Part model, mm, in its own coordinate system. Round coordinates to 2 decimals unless told otherwise and drop trailing zeros. Order: outer loops, then holes, each group sorted by start corner. A loop starts at its lowest first (then second) coordinate and runs counter-clockwise, first axis right, second up. Notation, with made-up numbers: (-15, 15) - (-9, 15) arc R31 ccw to (-9, 52) - close; hole circle Ø10 at (17.5, 35.25). An arc over 180 degrees is marked (long way). Return JSON: item names as keys, results as strings. Group by question number.
Item 1: Saw through at B-B on z = 0.9. State how many separate pieces and enclosed holes the cut face has, and give its area (3 significant figures).
Item 2: Saw through at A-A on x = 292. List the corners of the cut face in (y, z) (3 decimals), and give its area (3 significant figures).
Item 3: Drop flat-ended pins along their axis: pin 1 (1 mm diameter, centred on y = 36.5, z = 2, fed in from +X); pin 2 (6.5 mm diameter, centred on x = 660.4, y = 9.525, fed in from -Z). Give the stop position or say it passes through.
Item 4: Probe probe 1 along Y at (x, z) = (190.5, 1.4); probe 2 along Y at (x, z) = (469.9, 1.3); probe 3 along X at (y, z) = (43.5, 1.95). List the from-to ranges inside material, lowest first.
Item 5: Two-plate mould, pull along X, no slides. Class faces 1 (the face through (838.38, 19.32, 1.61)), 2 (the face through (431, 50, 0)), 3 (the face through (743.7, 40.3, 1.6)): released by +X, released by -X, zero draft, split by the parting line, or undercut.
Autodesk Inventor part; units mm, degrees
ref_plane "YZ Plane" through (0, 0, 0) normal (1, 0, 0) x (0, 1, 0)
ref_plane "XZ Plane" through (0, 0, 0) normal (0, 1, 0) x (-1, 0, 0)
ref_plane "XY Plane" through (0, 0, 0) normal (0, 0, 1) x (1, 0, 0)
sketch "Sketch1" plane through (0, 0, 0) normal (0, 0, 1) x (1, 0, 0)
  line L0 (0, 0) -> (850.9, 0)
  line L1 (850.9, 0) -> (850.9, 76.2)
  line L2 (850.9, 76.2) -> (0, 76.2)
  line L3 (0, 76.2) -> (0, 0)
  dimension "d0" = 850.9
  dimension "d1" = 76.2
extrude "Extrusion1" add sketch "Sketch1" along normal blind 3.175
sketch "Sketch4" plane through (0, 0, 3.175) normal (0, 0, 1) x (1, 0, 0)
  line L0 (0, 0) -> (0, 38.1)
  line L1 (0, 76.2) -> (0, 0)
  line L2 (0, 0) -> (25.4, 0)
  line L3 (0, 0) -> (850.9, 0)
  line L4 (25.4, 0) -> (0, 38.1)
  line L5 (850.9, 0) -> (825.5, 0)
  line L6 (850.9, 0) -> (850.9, 38.1)
  line L7 (850.9, 0) -> (850.9, 76.2)
  line L8 (850.9, 38.1) -> (825.5, 0)
  line L9 (0, 38.1) -> (0, 36.5125)
  circle A0 centre (292.9509, 36.5125) radius 14.2875
  circle A1 centre (557.9491, 36.5125) radius 14.2875
  circle A2 centre (757.9743, 39.6875) radius 14.2875
  circle A3 centre (92.9257, 39.6875) radius 14.2875
  dimension "d24" = 38.1
  dimension "d26" = 25.4
  dimension "d27" = 38.1
  dimension "d33" = 28.575
  dimension "d34" = 28.575
  dimension "d38" = 28.575
  dimension "d39" = 28.575
extrude "Extrusion3" cut sketch "Sketch4" against normal blind 3.175
sketch "Sketch5" plane through (0, 0, 3.175) normal (0, 0, 1) x (1, 0, 0)
  line L0 (850.9, 76.2) -> (0, 76.2)
  line L1 (0, 76.2) -> (425.45, 76.2)
  circle A0 centre (425.45, 66.675) radius 3.5687
  circle A1 centre (425.45, 9.525) radius 3.5687
  line L2 (25.4, 0) -> (825.5, 0)
  line L3 (0, 76.2) -> (190.5, 76.2)
  circle A2 centre (190.5, 66.675) radius 3.5687
  circle A3 centre (190.5, 9.525) radius 3.5687
  circle A4 centre (190.5, 38.1) radius 3.5687
  line L4 (850.9, 38.1) -> (850.9, 76.2)
  line L5 (850.9, 76.2) -> (660.4, 76.2)
  circle A5 centre (660.4, 66.675) radius 3.5687
  circle A6 centre (660.4, 9.525) radius 3.5687
  circle A7 centre (660.4, 38.1) radius 3.5687
  circle A8 centre (838.2, 63.5) radius 3.5687
  circle A9 centre (12.7, 63.5) radius 3.5687
  line L6 (0, 76.2) -> (0, 38.1)
  circle A10 centre (34.925, 12.7) radius 3.5687
  circle A11 centre (815.975, 12.7) radius 3.5687
  point P0 (0, 0)
  dimension "d42" = 425.45
  dimension "d43" = 7.1374
  dimension "d44" = 9.525
  dimension "d45" = 7.1374
  dimension "d46" = 9.525
  dimension "d47" = 190.5
  dimension "d48" = 7.1374
  dimension "d49" = 9.525
  dimension "d50" = 7.1374
  dimension "d51" = 9.525
  dimension "d52" = 7.1374
  dimension "d53" = 38.1
  dimension "d54" = 190.5
  dimension "d55" = 7.1374
  dimension "d56" = 9.525
  dimension "d57" = 7.1374
  dimension "d58" = 9.525
  dimension "d59" = 7.1374
  dimension "d60" = 38.1
  dimension "d61" = 7.1374
  dimension "d62" = 12.7
  dimension "d63" = 12.7
  dimension "d64" = 7.1374
  dimension "d65" = 12.7
  dimension "d66" = 12.7
  dimension "d67" = 7.1374
  dimension "d69" = 12.7
  dimension "d70" = 9.525
  dimension "d71" = 7.1374
  dimension "d72" = 12.7
  dimension "d73" = 9.525
extrude "Extrusion4" cut sketch "Sketch5" against normal blind 3.175
sketch "Sketch6" plane through (0, 0, 3.175) normal (0, 0, 1) x (1, 0, 0)
  circle A0 centre (361.95, 38.1) radius 3.5687
  circle A1 centre (469.9, 38.1) radius 3.5687
  line L0 (850.9, 76.2) -> (0, 76.2)
  circle A2 centre (292.9509, 36.5125) radius 14.2875
  line L1 (0, 76.2) -> (0, 38.1)
  line L2 (850.9, 38.1) -> (850.9, 76.2)
  point P0 (0, 0)
  dimension "d76" = 7.1374
  dimension "d77" = 7.1374
  dimension "d78" = 38.1
  dimension "d79" = 38.1
  dimension "d82" = 381
  dimension "d83" = 361.95
extrude "Extrusion6" cut sketch "Sketch6" against normal blind 25.4 contours A0 | A1
sketch "Sketch7" plane through (0, 76.2, 0) normal (0, 1, 0) x (1, 0, 0)
  line L0 (850.9, 0) -> (0, 0)
  line L1 (0, 0) -> (0, -3.175)
  line L2 (850.9, -3.175) -> (0, -3.175)
  line L3 (850.9, 0) -> (850.9, -3.175)
extrude "Extrusion7" add sketch "Sketch7" along normal blind 25.4
sketch "Sketch8" plane through (0, 0, 3.175) normal (0, 0, 1) x (1, 0, 0)
  circle A0 centre (12.7, 63.5) radius 3.5687
  circle A1 centre (838.2, 63.5) radius 3.5687
  circle A2 centre (425.45, 66.675) radius 3.5687
  point P0 (0, 0)
extrude "Extrusion9" add sketch "Sketch8" against normal blind 3.175
sketch "Sketch9" plane through (0, 0, 3.175) normal (0, 0, 1) x (1, 0, 0)
  circle A0 centre (12.7, 88.9) radius 3.5687
  line L0 (0, 101.6) -> (850.9, 101.6)
  line L1 (0, 38.1) -> (0, 101.6)
  circle A1 centre (838.2, 88.9) radius 3.5687
  line L2 (850.9, 38.1) -> (850.9, 101.6)
  circle A2 centre (425.45, 88.9) radius 3.5687
  point P0 (0, 0)
  dimension "d95" = 7.1374
  dimension "d96" = 12.7
  dimension "d97" = 12.7
  dimension "d98" = 7.1374
  dimension "d99" = 12.7
  dimension "d100" = 12.7
  dimension "d101" = 7.1374
extrude "Extrusion10" cut sketch "Sketch9" against normal blind 3.175
properties part number "OutsidePlate2" material "Aluminum 6061"
Filled in:
{
 "1": {"separate pieces": "1", "enclosed holes": "18", "area": "82,400 mm^2"},
 "2": {"outline": "(0, 0) - (22.257, 0) - (22.257, 3.175) - (0, 3.175) - close; (50.768, 0) - (101.6, 0) - (101.6, 3.175) - (50.768, 3.175) - close", "area": "232 mm^2"},
 "3": {"pin 1": "stops at x = 850.17", "pin 2": "passes through"},
 "4": {"probe 1": "y = 0 to 5.96, 13.09 to 34.53, 41.67 to 63.11, 70.24 to 101.6", "probe 2": "y = 0 to 34.53, 41.67 to 101.6", "probe 3": "x = 0 to 79.16, 106.7 to 280.49, 305.41 to 545.49, 570.41 to 744.2, 771.74 to 850.9"},
 "5": {"face 1": "released by +X", "face 2": "zero draft", "face 3": "undercut"}
}
